```python
from build123d import *

# Parameters (mm, degrees)
BOSS_EXTRUDE1_DEPTH = 5
BOSS_EXTRUDE2_DEPTH = 25
CUT_EXTRUDE1_REACH  = 32
SKETCH4_R           = 2.1
CUT_EXTRUDE2_REACH  = 27
BOSS_EXTRUDE4_DEPTH = 18.32
SKETCH9_R           = 1.25
CUT_EXTRUDE3_DEPTH  = 10
CUT_EXTRUDE4_REACH  = 32
SKETCH10_R          = 2.1


with BuildPart() as part:
    # Sketch1 → Boss-Extrude1 (new body)
    with BuildSketch(Plane.XY):
        with BuildLine():
            Line((-47.5, 70), (47.5, 70))
            ThreePointArc((47.5, 70), (51.035533906, 68.535533906), (52.5, 65))
            Line((52.5, 65), (52.5, -65))
            ThreePointArc((52.5, -65), (51.035533906, -68.535533906), (47.5, -70))
            Line((47.5, -70), (-47.5, -70))
            ThreePointArc((-47.5, -70), (-51.035533906, -68.535533906), (-52.5, -65))
            Line((-52.5, -65), (-52.5, 65))
            ThreePointArc((-52.5, 65), (-51.035533906, 68.535533906), (-47.5, 70))
        make_face()
        with BuildLine():
            Line((-32, 56.5), (32, 56.5))
            ThreePointArc((32, 56.5), (34.828427125, 55.328427125), (36, 52.5))
            Line((36, 52.5), (36, -52.5))
            ThreePointArc((36, -52.5), (34.828427125, -55.328427125), (32, -56.5))
            Line((32, -56.5), (-32, -56.5))
            ThreePointArc((-32, -56.5), (-34.828427125, -55.328427125), (-36, -52.5))
            Line((-36, -52.5), (-36, 52.5))
            ThreePointArc((-36, 52.5), (-34.828427125, 55.328427125), (-32, 56.5))
        make_face(mode=Mode.SUBTRACT)
    extrude(amount=BOSS_EXTRUDE1_DEPTH)

    # Sketch2 → Boss-Extrude2 (add)
    with BuildSketch(Plane(origin=(0, 0, 0), x_dir=(-1, 0, 0), z_dir=(0, 0, -1))):
        with BuildLine():
            Line((-33.5, 60), (33.5, 60))
            ThreePointArc((33.5, 60), (37.742640687, 58.242640687), (39.5, 54))
            Line((39.5, 54), (39.5, -54))
            ThreePointArc((39.5, -54), (37.742640687, -58.242640687), (33.5, -60))
            Line((33.5, -60), (-33.5, -60))
            ThreePointArc((-33.5, -60), (-37.742640687, -58.242640687), (-39.5, -54))
            Line((-39.5, -54), (-39.5, 54))
            ThreePointArc((-39.5, 54), (-37.742640687, 58.242640687), (-33.5, 60))
        make_face()
    extrude(amount=BOSS_EXTRUDE2_DEPTH)

    # Sketch4 → Cut-Extrude1 (cut, up to next)
    with BuildSketch(Plane.XY.offset(5), mode=Mode.PRIVATE) as cut_extrude1_sk1:
        with Locations((34.5, 65)):
            Circle(SKETCH4_R)
    cut_extrude1_tool1 = extrude(cut_extrude1_sk1.sketch, amount=-CUT_EXTRUDE1_REACH, mode=Mode.PRIVATE) & part.part
    add(cut_extrude1_tool1.solids().sort_by_distance((34.5, 65, 5))[0], mode=Mode.SUBTRACT)
    # Sketch4 → Cut-Extrude1 (cut, up to next)
    with BuildSketch(Plane.XY.offset(5), mode=Mode.PRIVATE) as cut_extrude1_sk2:
        with Locations((-34.5, 65)):
            Circle(SKETCH4_R)
    cut_extrude1_tool2 = extrude(cut_extrude1_sk2.sketch, amount=-CUT_EXTRUDE1_REACH, mode=Mode.PRIVATE) & part.part
    add(cut_extrude1_tool2.solids().sort_by_distance((-34.5, 65, 5))[0], mode=Mode.SUBTRACT)
    # Sketch4 → Cut-Extrude1 (cut, up to next)
    with BuildSketch(Plane.XY.offset(5), mode=Mode.PRIVATE) as cut_extrude1_sk3:
        with Locations((-34.5, -65)):
            Circle(SKETCH4_R)
    cut_extrude1_tool3 = extrude(cut_extrude1_sk3.sketch, amount=-CUT_EXTRUDE1_REACH, mode=Mode.PRIVATE) & part.part
    add(cut_extrude1_tool3.solids().sort_by_distance((-34.5, -65, 5))[0], mode=Mode.SUBTRACT)
    # Sketch4 → Cut-Extrude1 (cut, up to next)
    with BuildSketch(Plane.XY.offset(5), mode=Mode.PRIVATE) as cut_extrude1_sk4:
        with Locations((34.5, -65)):
            Circle(SKETCH4_R)
    cut_extrude1_tool4 = extrude(cut_extrude1_sk4.sketch, amount=-CUT_EXTRUDE1_REACH, mode=Mode.PRIVATE) & part.part
    add(cut_extrude1_tool4.solids().sort_by_distance((34.5, -65, 5))[0], mode=Mode.SUBTRACT)

    # Sketch5 → Cut-Extrude2 (cut, up to next)
    with BuildSketch(Plane.XY, mode=Mode.PRIVATE) as cut_extrude2_sk1:
        with BuildLine():
            Line((-32, 56.5), (32, 56.5))
            ThreePointArc((32, 56.5), (34.828427125, 55.328427125), (36, 52.5))
            Line((36, 52.5), (36, -52.5))
            ThreePointArc((36, -52.5), (34.828427125, -55.328427125), (32, -56.5))
            Line((32, -56.5), (-32, -56.5))
            ThreePointArc((-32, -56.5), (-34.828427125, -55.328427125), (-36, -52.5))
            Line((-36, -52.5), (-36, 52.5))
            ThreePointArc((-36, 52.5), (-34.828427125, 55.328427125), (-32, 56.5))
        make_face()
    cut_extrude2_tool1 = extrude(cut_extrude2_sk1.sketch, amount=-CUT_EXTRUDE2_REACH, mode=Mode.PRIVATE) & part.part
    add(cut_extrude2_tool1.solids().sort_by_distance((0, 0, 0))[0], mode=Mode.SUBTRACT)

    # Sketch8 → Boss-Extrude4 (add)
    with BuildSketch(Plane(origin=(0, 0, -25), x_dir=(-1, 0, 0), z_dir=(0, 0, -1))):
        with BuildLine():
            Line((-28.25, 52.25), (-28.25, 56.5))
            Line((-28.25, 56.5), (-32, 56.5))
            ThreePointArc((-32, 56.5), (-34.828427125, 55.328427125), (-36, 52.5))
            Line((-36, 52.5), (-36, 49.25))
            Line((-36, 49.25), (-31.25, 49.25))
            ThreePointArc((-31.25, 49.25), (-29.128679656, 50.128679656), (-28.25, 52.25))
        make_face()
        with BuildLine():
            Line((0, 49.25), (0, 56.5))
            Line((0, 56.5), (-7.75, 56.5))
            Line((-7.75, 56.5), (-7.75, 52.25))
            ThreePointArc((-7.75, 52.25), (-6.871320344, 50.128679656), (-4.75, 49.25))
            Line((-4.75, 49.25), (0, 49.25))
        make_face()
        with BuildLine():
            Line((7.75, 52.25), (7.75, 56.5))
            Line((7.75, 56.5), (0, 56.5))
            Line((0, 56.5), (0, 49.25))
            Line((0, 49.25), (4.75, 49.25))
            ThreePointArc((4.75, 49.25), (6.871320344, 50.128679656), (7.75, 52.25))
        make_face()
        with BuildLine():
            Line((28.25, 56.5), (28.25, 52.25))
            ThreePointArc((28.25, 52.25), (29.128679656, 50.128679656), (31.25, 49.25))
            Line((31.25, 49.25), (36, 49.25))
            Line((36, 49.25), (36, 52.5))
            ThreePointArc((36, 52.5), (34.828427125, 55.328427125), (32, 56.5))
            Line((32, 56.5), (28.25, 56.5))
        make_face()
        with BuildLine():
            Line((-31.25, -49.25), (-36, -49.25))
            Line((-36, -49.25), (-36, -52.5))
            ThreePointArc((-36, -52.5), (-34.828427125, -55.328427125), (-32, -56.5))
            Line((-32, -56.5), (-28.25, -56.5))
            Line((-28.25, -56.5), (-28.25, -52.25))
            ThreePointArc((-28.25, -52.25), (-29.128679656, -50.128679656), (-31.25, -49.25))
        make_face()
        with BuildLine():
            Line((-7.75, -56.5), (0, -56.5))
            Line((0, -56.5), (0, -49.25))
            Line((0, -49.25), (-4.75, -49.25))
            ThreePointArc((-4.75, -49.25), (-6.871320344, -50.128679656), (-7.75, -52.25))
            Line((-7.75, -52.25), (-7.75, -56.5))
        make_face()
        with BuildLine():
            Line((0, -56.5), (7.75, -56.5))
            Line((7.75, -56.5), (7.75, -52.25))
            ThreePointArc((7.75, -52.25), (6.871320344, -50.128679656), (4.75, -49.25))
            Line((4.75, -49.25), (0, -49.25))
            Line((0, -49.25), (0, -56.5))
        make_face()
        with BuildLine():
            Line((36, -52.5), (36, -49.25))
            Line((36, -49.25), (31.25, -49.25))
            ThreePointArc((31.25, -49.25), (29.128679656, -50.128679656), (28.25, -52.25))
            Line((28.25, -52.25), (28.25, -56.5))
            Line((28.25, -56.5), (32, -56.5))
            ThreePointArc((32, -56.5), (34.828427125, -55.328427125), (36, -52.5))
        make_face()
    extrude(amount=-BOSS_EXTRUDE4_DEPTH)

    # Sketch9 → Cut-Extrude3 (cut)
    with BuildSketch(Plane.XY.offset(-6.68)):
        with Locations((-4.5, 52)):
            Circle(SKETCH9_R)
        with Locations((-31.5, 52)):
            Circle(SKETCH9_R)
        with Locations((31.5, 52)):
            Circle(SKETCH9_R)
        with Locations((4.5, 52)):
            Circle(SKETCH9_R)
        with Locations((4.5, -52)):
            Circle(SKETCH9_R)
        with Locations((31.5, -52)):
            Circle(SKETCH9_R)
        with Locations((-31.5, -52)):
            Circle(SKETCH9_R)
        with Locations((-4.5, -52)):
            Circle(SKETCH9_R)
    extrude(amount=-CUT_EXTRUDE3_DEPTH, mode=Mode.SUBTRACT)

    # Sketch10 → Cut-Extrude4 (cut, up to next)
    with BuildSketch(Plane.XY.offset(5), mode=Mode.PRIVATE) as cut_extrude4_sk1:
        with Locations((-46, 57)):
            Circle(SKETCH10_R)
    cut_extrude4_tool1 = extrude(cut_extrude4_sk1.sketch, amount=-CUT_EXTRUDE4_REACH, mode=Mode.PRIVATE) & part.part
    add(cut_extrude4_tool1.solids().sort_by_distance((-46, 57, 5))[0], mode=Mode.SUBTRACT)
    # Sketch10 → Cut-Extrude4 (cut, up to next)
    with BuildSketch(Plane.XY.offset(5), mode=Mode.PRIVATE) as cut_extrude4_sk2:
        with Locations((46, 57)):
            Circle(SKETCH10_R)
    cut_extrude4_tool2 = extrude(cut_extrude4_sk2.sketch, amount=-CUT_EXTRUDE4_REACH, mode=Mode.PRIVATE) & part.part
    add(cut_extrude4_tool2.solids().sort_by_distance((46, 57, 5))[0], mode=Mode.SUBTRACT)
    # Sketch10 → Cut-Extrude4 (cut, up to next)
    with BuildSketch(Plane.XY.offset(5), mode=Mode.PRIVATE) as cut_extrude4_sk3:
        with Locations((46, -57)):
            Circle(SKETCH10_R)
    cut_extrude4_tool3 = extrude(cut_extrude4_sk3.sketch, amount=-CUT_EXTRUDE4_REACH, mode=Mode.PRIVATE) & part.part
    add(cut_extrude4_tool3.solids().sort_by_distance((46, -57, 5))[0], mode=Mode.SUBTRACT)
    # Sketch10 → Cut-Extrude4 (cut, up to next)
    with BuildSketch(Plane.XY.offset(5), mode=Mode.PRIVATE) as cut_extrude4_sk4:
        with Locations((-46, -57)):
            Circle(SKETCH10_R)
    cut_extrude4_tool4 = extrude(cut_extrude4_sk4.sketch, amount=-CUT_EXTRUDE4_REACH, mode=Mode.PRIVATE) & part.part
    add(cut_extrude4_tool4.solids().sort_by_distance((-46, -57, 5))[0], mode=Mode.SUBTRACT)


solid = part.part
```
Check sheet for the modelled part. Datum: model origin and axes. Units: mm. A direction names the side the tool comes from. Round coordinates to 2 decimals unless told otherwise and drop trailing zeros. Order: outer loops, then holes, each group sorted by start corner. A loop starts at its lowest first (then second) coordinate and runs counter-clockwise, first axis right, second up. Notation, with made-up numbers: (20, -0.75) - (60, -0.75) arc R17 ccw to (60, 14.25) - close; hole circle Ø6 at (-14.75, 26). An arc over 180 degrees is marked (long way). Answer as CSV lines item,"result". Start each with the question number.
1) Section check C-C (z = -3.75). Record the cut outline in (x, y), then the cut area to 3 significant figures.
2) Scan lines: probe 1 along Y at (x, z) = (-46, 1.95); probe 2 along Y at (x, z) = (-4.5, -14); probe 3 along X at (y, z) = (40, 2.5). Record each from-to range of solid material in increasing order.
3) Section check B-B (x = -46). Record the cut outline in (y, z), then the cut area to 3 significant figures.
4) Depth check by flat-ended pin: pin 1 (12.5 mm diameter, centred on x = -6, z = -8.5, fed in from +Y); pin 2 (2 mm diameter, centred on y = -55, z = -16, fed in from +X); pin 3 (5 mm diameter, centred on x = 33.5, z = -12.5, fed in from -Y). Enter the tip coordinate at first touch or a pass-through.
5) Tool access check on faces 1 (the face through (37.789, 58.196, -12.325)), 2 (the face through (6.85, -50.11, -15.97)), 3 (the face through (34.797, 55.359, -0.758)). Record the directions out of +Z, -Z, +X, -X, +Y, -Y that give a thin tool (end or side, any length) a straight path to the whole face; none if there is none.
6) Section check D-D (z = -12.5). Give the number of separate pieces and of enclosed holes in the cut face, then the cut area to 3 significant figures.
7) Draft check along Y on faces 4 (the face through (-1, 70, 2)), 5 (the face through (-36.166, 63.722, 2.535)), 6 (the face through (37.696, -58.289, -12.325)). Enter one of: +Y half, -Y half, draft (parallel to the pull), parting line (faces both ways), or undercut.
8) Section check A-A (y = 15). Record the cut outline in (x, z).
Determined:
1,outline,"(-39.5, -54) arc R6 ccw to (-33.5, -60) - (33.5, -60) arc R6 ccw to (39.5, -54) - (39.5, 54) arc R6 ccw to (33.5, 60) - (-33.5, 60) arc R6 ccw to (-39.5, 54) - close; hole (-36, -52.5) arc R4 ccw to (-32, -56.5) - (32, -56.5) arc R4 ccw to (36, -52.5) - (36, 52.5) arc R4 ccw to (32, 56.5) - (-32, 56.5) arc R4 ccw to (-36, 52.5) - close"
1,area,"1,330 mm^2"
2,probe 1,"-70 to -59.1, -54.9 to 54.9, 59.1 to 70"
2,probe 2,"-60 to -53.25, -50.75 to -49.25, 49.25 to 50.75, 53.25 to 60"
2,probe 3,"-52.5 to -36, 36 to 52.5"
3,outline,"(-70, 0) - (-59.1, 0) - (-59.1, 5) - (-70, 5) - close; (-54.9, 0) - (54.9, 0) - (54.9, 5) - (-54.9, 5) - close; (59.1, 0) - (70, 0) - (70, 5) - (59.1, 5) - close"
3,area,"658 mm^2"
4,pin 1,"y = 60"
4,pin 2,"x = 39.5"
4,pin 3,"y = -60"
5,face 1,"-Z, +X, +Y"
5,face 2,"+Z, -Z"
5,face 3,"+Z"
6,separate pieces,"1"
6,enclosed holes,"9"
6,area,"1,710 mm^2"
7,face 4,"+Y half"
7,face 5,"undercut"
7,face 6,"-Y half"
8,outline,"(-52.5, 0) - (-39.5, 0) - (-39.5, -25) - (-36, -25) - (-36, 5) - (-52.5, 5) - close; (36, -25) - (39.5, -25) - (39.5, 0) - (52.5, 0) - (52.5, 5) - (36, 5) - close"
